Check sheet for the drawn part. Datum: minimum x, y, z corner. Units: mm. Round coordinates to 2 decimals unless told otherwise and drop trailing zeros. Write each loop counter-clockwise with the first axis right and the second up, starting at its lowest first coordinate (ties: lowest second). Pieces come first, ordered by that corner, then holes. Notation, with made-up numbers: (2, 31) -> (55, 31) arc R27 ccw to (55, 69) -> close; hole circle Ø5 at (48.25, 1.25). An arc over 180 degrees is marked (long way). Use CSV: the item, a comma, the result in double quotes.
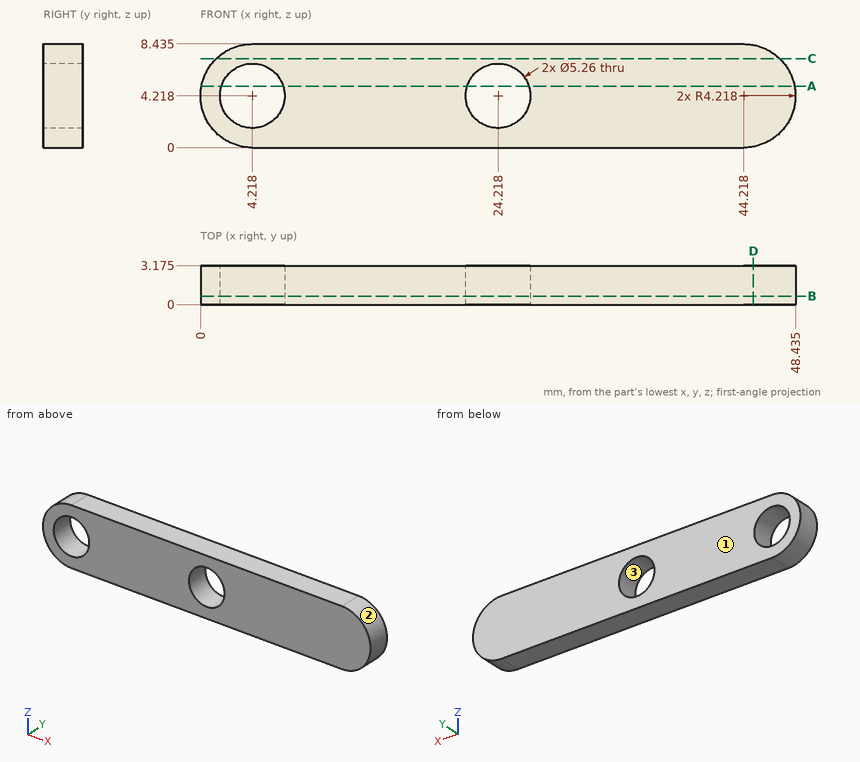
Q1. Mould release check, pull along X, two halves, no side actions. Record for the marked faces 1, 2 and 3: released by +X, released by -X, zero draft, split by the parting line, or undercut.
Filled in:
face 1,"zero draft"
face 2,"released by +X"
face 3,"undercut"
Q2. Go/stop test with a flat-tipped pin: P1, Ø1.5, axis at y = 2, z = 2.5, coming from the -X side. Record where the tip stops, or that it passes through.
Filled in:
P1,"x = 0.11"
Q3. Section check A-A (z = 5). Record the cut outline in (x, y) (1 decimal).
Filled in:
outline,"(0.1, 0) -> (1.7, 0) -> (1.7, 3.2) -> (0.1, 3.2) -> close; (6.7, 0) -> (21.7, 0) -> (21.7, 3.2) -> (6.7, 3.2) -> close; (26.7, 0) -> (48.4, 0) -> (48.4, 3.2) -> (26.7, 3.2) -> close"
Q4. Material ranges on L1, parallel to X at y = 1.9, z = 4 (1 decimal); L2, parallel to X at y = 1.5, z = 2.75 (1 decimal); L3, parallel to Z at x = 25.5, y = 0.75 (1 decimal), recorded low to high.
Filled in:
L1,"0 to 1.6, 6.8 to 21.6, 26.8 to 48.4"
L2,"0.3 to 2, 6.4 to 22, 26.4 to 48.2"
L3,"0 to 1.9, 6.5 to 8.4"
Q5. Section check C-C (z = 7.25). Record the cut outline in (x, y) (1 decimal).
Filled in:
outline,"(1.3, 0) -> (47.1, 0) -> (47.1, 3.2) -> (1.3, 3.2) -> close"
Q6. Section check B-B (y = 0.7). Record the cut outline in (x, z) (1 decimal).
Filled in:
outline,"(4.2, 0) -> (44.2, 0) arc R4.2 ccw to (44.2, 8.4) -> (4.2, 8.4) arc R4.2 ccw to start; hole circle Ø5.3 at (4.2, 4.2); hole circle Ø5.3 at (24.2, 4.2)"
Q7. Section check D-D (x = 45). Record the cut outline in (y, z) (1 decimal), plus the area to 3 significant figures.
Filled in:
outline,"(0, 0.1) -> (3.2, 0.1) -> (3.2, 8.4) -> (0, 8.4) -> close"
area,"26.3 mm²"
